from build123d import *

# Parameters (mm, degrees)
SKETCH1_W           = 100.6
SKETCH1_H           = 100.6
BOSS_EXTRUDE1_DEPTH = 113
SKETCH2_W           = 10
SKETCH2_H           = 10
BOSS_EXTRUDE2_DEPTH = 5
SKETCH3_W           = 10
SKETCH3_H           = 10
BOSS_EXTRUDE3_DEPTH = 5


with BuildPart() as part:
    # Sketch1 → Boss-Extrude1 (new, symmetric)
    with BuildSketch(Plane.XY):
        Rectangle(SKETCH1_W, SKETCH1_H)
    extrude(amount=BOSS_EXTRUDE1_DEPTH, both=True)

    # Sketch2 → Boss-Extrude2 (add)
    with BuildSketch(Plane.XY.offset(113)):
        with Locations((-45.3, 45.3)):
            Rectangle(SKETCH2_W, SKETCH2_H)
        with Locations((45.3, 45.3)):
            Rectangle(SKETCH2_W, SKETCH2_H)
        with Locations((45.3, -45.3)):
            Rectangle(SKETCH2_W, SKETCH2_H)
        with Locations((-45.3, -45.3)):
            Rectangle(SKETCH2_W, SKETCH2_H)
    extrude(amount=BOSS_EXTRUDE2_DEPTH)

    # Sketch3 → Boss-Extrude3 (add)
    with BuildSketch(Plane(origin=(0, 0, -113), x_dir=(-1, 0, 0), z_dir=(0, 0, -1))):
        with Locations((-45.3, 45.3)):
            Rectangle(SKETCH3_W, SKETCH3_H)
        with Locations((45.3, 45.3)):
            Rectangle(SKETCH3_W, SKETCH3_H)
        with Locations((45.3, -45.3)):
            Rectangle(SKETCH3_W, SKETCH3_H)
        with Locations((-45.3, -45.3)):
            Rectangle(SKETCH3_W, SKETCH3_H)
    extrude(amount=BOSS_EXTRUDE3_DEPTH)


solid = part.part
Part model, mm, in its own coordinate system. A direction names the side the tool comes from. Coordinates: 2 decimals unless noted, no trailing zeros. Order: outer loops, then holes, each group sorted by start corner. A loop starts at its lowest first (then second) coordinate and runs counter-clockwise, first axis right, second up.
(1) Slice it at A-A, the plane y = -43. Write the cut outline in (x, z).
Check sheet entries:
outline: (-50.3, -118) - (-40.3, -118) - (-40.3, -113) - (40.3, -113) - (40.3, -118) - (50.3, -118) - (50.3, 118) - (40.3, 118) - (40.3, 113) - (-40.3, 113) - (-40.3, 118) - (-50.3, 118) - close
(2) Pin check, flat tips, straight feed: pin 1 Ø1 at (x, y) = (4, 26) entering from +Z; pin 2 Ø5 at (x, y) = (-4.5, 2.5) entering from -Z. Stop position of each tip, or through.
Check sheet entries:
pin 1: stops at z = 113
pin 2: stops at z = -113
(3) Probe L1, parallel to Z at x = -11, y = -44.5. List the from-to ranges inside material, lowest first.
Check sheet entries:
L1: z = -113 to 113
(4) Tool access for faces 1 (the face through (45, 40.3, 115)), 2 (the face through (45, -45, 118)), 3 (the face through (-40.3, 45, 115)), 4 (the face through (-45, 45, -118)), 5 (the face through (-45, -40.3, -115)): list every direction of +Z, -Z, +X, -X, +Y, -Y with a clear straight run to the whole face (end or side of a thin tool).
Check sheet entries:
face 1: +Z, +X, -X
face 2: +Z, +X, -X, +Y, -Y
face 3: +Z, +Y, -Y
face 4: -Z, +X, -X, +Y, -Y
face 5: -Z, +X, -X
(5) Pull direction X, two halves, no side cores. Call faces 6 (the face through (-1, -50.3, 2)), 7 (the face through (-40.3, 45, -115)), 8 (the face through (50.3, -1, 2)): pulls with the +X half, pulls with the -X half, needs draft (parallel to the pull), parting line crosses it, or undercut.
Check sheet entries:
face 6: needs draft
face 7: undercut
face 8: pulls with the +X half
(6) Slice it at C-C, the plane y = -3.5. Write the cut outline in (x, z).
Check sheet entries:
outline: (-50.3, -113) - (50.3, -113) - (50.3, 113) - (-50.3, 113) - close
